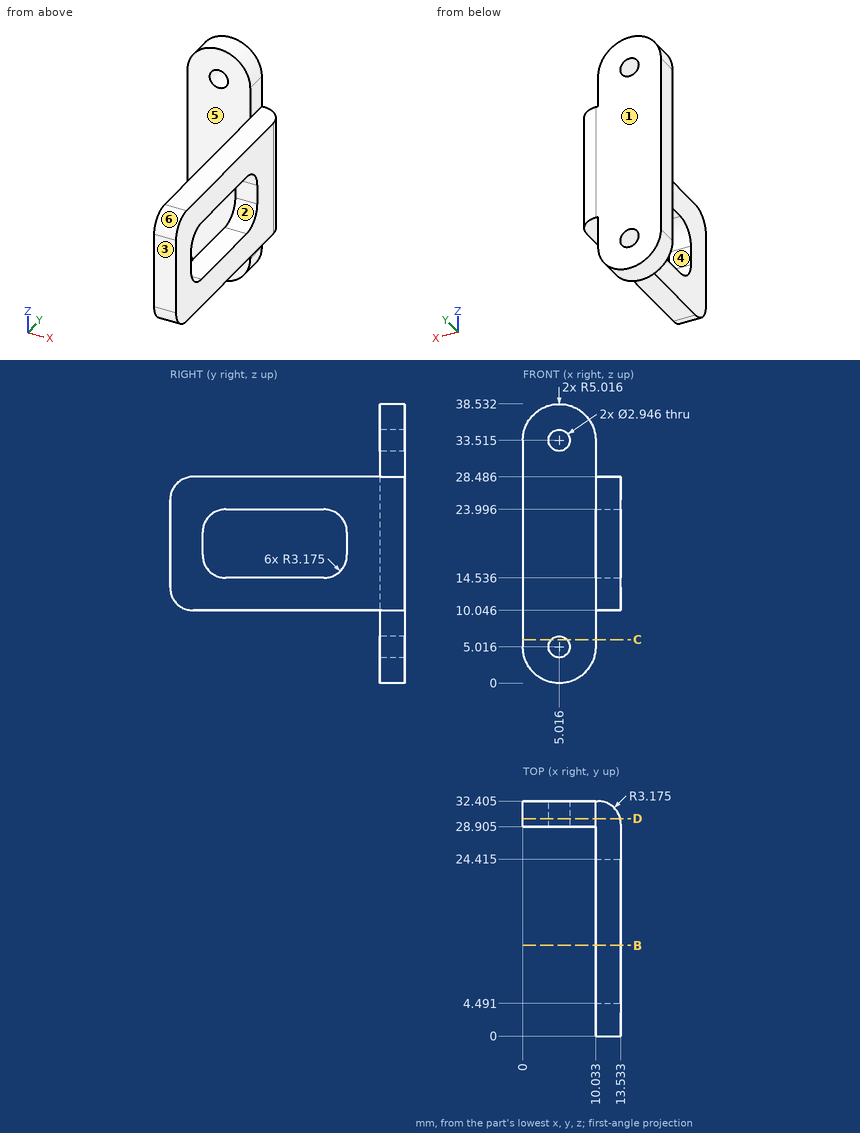
Here's the drawing with two shaded views (mm, measured from the low corner). I have some questions. A direction names the side the tool comes from. Coordinates: 2 decimals unless noted, no trailing zeros. Order: outer loops, then holes, each group sorted by start corner. A loop starts at its lowest first (then second) coordinate and runs counter-clockwise, first axis right, second up.
Q1. Suppose I cut it at D-D on y = 30. Please give me the cut outline in (x, z) (1 decimal).
Q2. Will these pins go through, and if not, where does the flat tip stop? pin 1 (9 mm diameter, centred on y = 10.5, z = 21.5, fed in from -X); pin 2 (3 mm diameter, centred on x = 7, z = 27.5, fed in from -Y) (1 decimal); pin 3 (4 mm diameter, centred on y = 31, z = 6.5, fed in from +X); pin 4 (6 mm diameter, centred on y = 20, z = 7, fed in from -X).
Q3. Thinking about a two-plate mould opening in Y: for the marked faces 1, 2 and 3, which applies, released by +Y, released by -Y, zero draft, split by the parting line, or undercut?
Q4. Please list where these lines run through material, in increasing order: L1, parallel to Z at x = 10.25, y = 13.5 (1 decimal); L2, parallel to Z at x = 11.25, y = 28 (1 decimal); L3, parallel to X at y = 16.5, z = 12.5.
Q5. Suppose I cut it at C-C on z = 6. Please give me the cut outline in (x, y) (1 decimal).
Q6. Which directions (+Z, -Z, +X, -X, +Y, -Y) give clear straight access to the entire face, cutting with the end or side of a thin tool? Please do the marked faces 4, 5 and 6.
Q7. Suppose I cut it at B-B on y = 12.5. Please give me the cut outline in (x, z) (1 decimal).
Answer:
1. outline: (0, 5) arc R5 ccw to (10, 5) - (10, 10) - (13.4, 10) - (13.4, 28.5) - (10, 28.5) - (10, 33.5) arc R5 ccw to (0, 33.5) - close; hole circle Ø2.9 at (5, 5); hole circle Ø2.9 at (5, 33.5)
2. pin 1: stops at x = 10.03
2. pin 2: stops at y = 28.9
2. pin 3: stops at x = 10.03
2. pin 4: passes through
3. face 1: released by +Y
3. face 2: undercut
3. face 3: released by -Y
4. L1: z = 10 to 14.5, 24 to 28.5
4. L2: z = 10 to 28.5
4. L3: x = 10.03 to 13.53
5. outline: (0, 28.9) - (3.9, 28.9) - (3.9, 32.4) - (0, 32.4) - close; (6.1, 28.9) - (10, 28.9) - (10, 32.4) - (6.1, 32.4) - close
6. face 4: +X, -X
6. face 5: +Z, -Z, -X, -Y
6. face 6: +Z, +X, -X, -Y
7. outline: (10, 10) - (13.5, 10) - (13.5, 14.5) - (10, 14.5) - close; (10, 24) - (13.5, 24) - (13.5, 28.5) - (10, 28.5) - close
